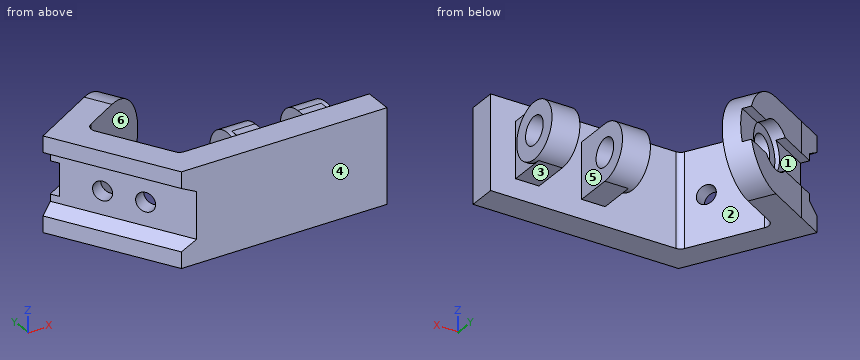
```python
from build123d import *

# Parameters (mm, degrees)
BOSS_EXTRUDE1_DEPTH = 64
SKETCH2_R           = 9.5
BOSS_EXTRUDE3_DEPTH = 18
CUT_EXTRUDE1_DEPTH  = 128
SKETCH4_W           = 79.210461268
SKETCH4_H           = 22
CUT_EXTRUDE2_DEPTH  = 6
SKETCH5_R           = 16
CUT_EXTRUDE4_DEPTH  = 9
SKETCH6_R           = 6.5
CUT_EXTRUDE6_DEPTH  = 10
FILLET1_R           = 5
FILLET2_R           = 6
SKETCH7_W           = 16
SKETCH7_H           = 38
BOSS_EXTRUDE4_DEPTH = 25
SKETCH8_R           = 19
SKETCH8_R_2         = 9.5
BOSS_EXTRUDE5_DEPTH = 19
SKETCH9_R           = 9.5
CUT_EXTRUDE7_DEPTH  = 19
SKETCH11_R          = 9.5
CUT_EXTRUDE8_DEPTH  = 19


with BuildPart() as part:
    # Sketch1 → Boss-Extrude1 (new body)
    with BuildSketch(Plane.XY):
        Polygon((-70, -9.5), (-115, 68.442286341), (-98.545517328, 77.942286341), (-59.030344885, 9.5), (70, 9.5), (70, -9.5), align=None)
    extrude(amount=BOSS_EXTRUDE1_DEPTH)

    # Sketch2 → Boss-Extrude3 (add)
    with BuildSketch(Plane(origin=(-58.386379332, 101.128175473, 0), x_dir=(0.866025404, 0.5, 0), z_dir=(-0.5, 0.866025404, 0))):
        with BuildLine():
            Line((-46.371778265, 0), (-46.371778265, -64))
            Line((-46.371778265, -64), (-14.371778265, -64))
            ThreePointArc((-14.371778265, -64), (17.628221735, -32), (-14.371778265, 0))
            Line((-14.371778265, 0), (-46.371778265, 0))
        make_face()
        with Locations((-14.371778265, -32)):
            Circle(SKETCH2_R, mode=Mode.SUBTRACT)
    extrude(amount=-BOSS_EXTRUDE3_DEPTH)

    # Sketch3 → Cut-Extrude1 (cut)
    with BuildSketch(Plane(origin=(-58.386379332, 101.128175473, 0), x_dir=(0.866025404, 0.5, 0), z_dir=(-0.5, 0.866025404, 0))):
        Polygon((-56.371778265, -16.196152423), (-56.371778265, -47.803847577), (-65.371778265, -53), (-65.371778265, -11), align=None)
    extrude(amount=-CUT_EXTRUDE1_DEPTH, mode=Mode.SUBTRACT)

    # Sketch4 → Cut-Extrude2 (cut)
    with BuildSketch(Plane(origin=(-58.386379332, 101.128175473, 0), x_dir=(0.866025404, 0.5, 0), z_dir=(-0.5, 0.866025404, 0))):
        with Locations((-20.439118131, -32)):
            Rectangle(SKETCH4_W, SKETCH4_H)
    extrude(amount=-CUT_EXTRUDE2_DEPTH, mode=Mode.SUBTRACT)

    # Sketch5 → Cut-Extrude4 (cut)
    with BuildSketch(Plane(origin=(-58.386379332, 101.128175473, 0), x_dir=(0.866025404, 0.5, 0), z_dir=(-0.5, 0.866025404, 0))):
        with Locations((-14.371778265, -32)):
            Circle(SKETCH5_R)
    extrude(amount=-CUT_EXTRUDE4_DEPTH, mode=Mode.SUBTRACT)

    # Sketch6 → Cut-Extrude6 (cut)
    with BuildSketch(Plane(origin=(-48.819392034, -28.185889132, 0), x_dir=(0, 0, 1), z_dir=(-0.866025404, -0.5, 0))):
        with Locations((32, 82.772758664)):
            Circle(SKETCH6_R)
        with Locations((32, 54.772758664)):
            Circle(SKETCH6_R)
    extrude(amount=-CUT_EXTRUDE6_DEPTH, mode=Mode.SUBTRACT)

    # Fillet1
    fillet1_edges = [part.edges().sort_by_distance(p)[0] for p in [
        (-59.030344885, 9.5, 32),
    ]]
    fillet(fillet1_edges, radius=FILLET1_R)

    # Fillet2
    fillet2_edges = [part.edges().sort_by_distance(p)[0] for p in [
        (-89.545517328, 62.353829072, 32),
    ]]
    fillet(fillet2_edges, radius=FILLET2_R)

    # Sketch7 → Boss-Extrude4 (add)
    with BuildSketch(Plane(origin=(0, 9.5, 0), x_dir=(1, 0, 0), z_dir=(0, 1, 0))):
        with Locations((45, -32)):
            Rectangle(SKETCH7_W, SKETCH7_H)
    boss_extrude4 = extrude(amount=BOSS_EXTRUDE4_DEPTH)

    # Sketch8 → Boss-Extrude5 (add)
    with BuildSketch(Plane(origin=(56, 0, 0), x_dir=(0, 0, -1), z_dir=(1, 0, 0))):
        with Locations((-32, 34.5)):
            Circle(SKETCH8_R)
        with Locations((-32, 34.5)):
            Circle(SKETCH8_R_2, mode=Mode.SUBTRACT)
    boss_extrude5 = extrude(amount=-BOSS_EXTRUDE5_DEPTH)

    # Sketch9 → Cut-Extrude7 (cut)
    with BuildSketch(Plane(origin=(56, 0, 0), x_dir=(0, 0, -1), z_dir=(1, 0, 0))):
        with Locations((-32, 34.5)):
            Circle(SKETCH9_R)
    extrude(amount=-CUT_EXTRUDE7_DEPTH, mode=Mode.SUBTRACT)

    # Mirror1: Boss-Extrude4, Boss-Extrude5 across plane
    add(boss_extrude4.mirror(Plane(origin=(22.5, 0, 0), x_dir=(0, 0, 1), z_dir=(1, 0, 0))))
    add(boss_extrude5.mirror(Plane(origin=(22.5, 0, 0), x_dir=(0, 0, 1), z_dir=(1, 0, 0))))

    # Sketch11 → Cut-Extrude8 (cut)
    with BuildSketch(Plane.ZY.offset(11)):
        with Locations((32, 34.5)):
            Circle(SKETCH11_R)
    extrude(amount=-CUT_EXTRUDE8_DEPTH, mode=Mode.SUBTRACT)


solid = part.part
```
Geometry check sheet. Reference: the model listing, model coordinates, mm. Face numbers are marked on the shaded views. A direction names the side the tool comes from. Coordinates: 2 decimals unless noted, no trailing zeros. Write each loop counter-clockwise with the first axis right and the second up, starting at its lowest first coordinate (ties: lowest second). Pieces come first, ordered by that corner, then holes. Notation, with made-up numbers: M -14,87 L 16,87 A14 ccw 16,96 Z; hole C 52.25,-13 d9. An arc over 180 degrees is marked long. Answer as a JSON object with one key per item and string values.
1. Go/stop test with flat-tipped pins: pin 1 Ø19 at (y, z) = (37.5, 36.5) entering from +X; pin 2 Ø19 at (y, z) = (28, 38) entering from -X; pin 3 Ø6 at (x, y) = (-50.5, 95.5) entering from +Z. Record where each tip stops, or that it passes through.
Answers below:
{"pin 1": "stops at x = 56", "pin 2": "stops at x = -86.74", "pin 3": "stops at z = 60.06"}
2. Draft check along X on the marked faces 4, 5 and 6. Enter one of: released by +X, released by -X, zero draft, split by the parting line, or undercut.
Answers below:
{"face 4": "zero draft", "face 5": "undercut", "face 6": "released by +X"}
3. Scan lines: L1, parallel to Y at x = 42.25, z = 32; L2, parallel to Z at x = -6.5, y = 34.5; L3, parallel to X at y = 23, z = 17. Record each from-to range of solid material in increasing order.
Answers below:
{"L1": "y = -9.5 to 25, 44 to 53.5", "L2": "z = 13 to 22.5, 41.5 to 51", "L3": "x = -78.37 to -66.82, -11 to 8, 37 to 56"}
4. Section check B-B, the plane z = 28.5. Give the number of separate pieces and of enclosed holes in the cut face, plus the area to 3 significant figures.
Answers below:
{"separate pieces": "6", "enclosed holes": "0", "area": "4,520 mm²"}
5. Tool access check on the marked faces 1, 2 and 3. Record the directions out of +Z, -Z, +X, -X, +Y, -Y that give a thin tool (end or side, any length) a straight path to the whole face; none if there is none.
Answers below:
{"face 1": "-X, +Y", "face 2": "+Z, -Z", "face 3": "-Z, +X, +Y"}
6. Section check C-C, the plane y = 2. Enter the section's corners in (x, z), plus the area to 3 significant figures.
Answers below:
{"outline": "M -76.64,0 L 70,0 L 70,64 L -76.64,64 L -76.64,53 L -66.25,47.8 L -66.25,16.2 L -76.64,11 Z", "area": "9,000 mm²"}
7. Section check A-A, the plane x = 43. Enter the section's corners in (y, z), plus the area to 3 significant figures.
Answers below:
{"outline": "M -9.5,0 L 9.5,0 L 9.5,13 L 34.5,13 A19 ccw 34.5,51 L 9.5,51 L 9.5,64 L -9.5,64 Z; hole C 34.5,32 d19", "area": "2,450 mm²"}
